Here's how the part is built. I have some questions about the finished solid (model axes, mm). Give positions to 0.01 mm unless a question says otherwise; leave off trailing zeros. Write each loop counter-clockwise with the first axis right and the second up, starting at its lowest first coordinate (ties: lowest second). Pieces come first, ordered by that corner, then holes. Notation, with made-up numbers: (76.25, 89.5) -> (110.25, 89.5) arc R23 cw to (110.25, 117.5) -> close; hole circle Ø5 at (-34, 16). An arc over 180 degrees is marked (long way). Return JSON: item names as keys, results as strings.
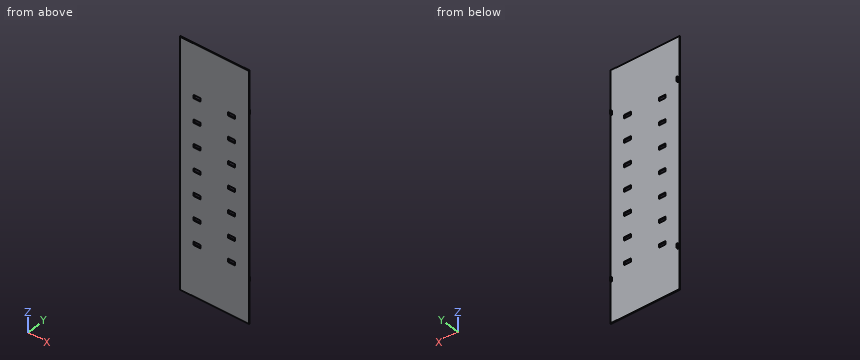
Solid Edge part; units mm, degrees
sketch "Sketch1" plane through (0, 0, 0) normal (0, -1, 0) x (1, 0, 0)
  line L0 (-254, -920.6611) -> (254, -920.6611)
  line L1 (254, -920.6611) -> (254, 920.6611)
  line L2 (254, 920.6611) -> (-254, 920.6611)
  line L3 (-254, 920.6611) -> (-254, -920.6611)
extrude "Protrusion1" add sketch "Sketch1" along normal mid plane 6.35
sketch "Sketch2" plane through (0, 3.175, 0) normal (0, 1, 0) x (-1, 0, 0)
  line L0 (-241.3, 590.4611) -> (-241.3, 622.2111)
  line L1 (-241.3, 622.2111) -> (-247.65, 622.2111)
  line L2 (-247.65, 622.2111) -> (-247.65, 590.4611)
  line L3 (-247.65, 590.4611) -> (-241.3, 590.4611)
  line L4 (241.3, 590.4611) -> (241.3, 622.2111)
  line L5 (241.3, 622.2111) -> (247.65, 622.2111)
  line L6 (247.65, 622.2111) -> (247.65, 590.4611)
  line L7 (247.65, 590.4611) -> (241.3, 590.4611)
  line L8 (-241.3, -590.4611) -> (-241.3, -622.2111)
  line L9 (-241.3, -622.2111) -> (-247.65, -622.2111)
  line L10 (-247.65, -622.2111) -> (-247.65, -590.4611)
  line L11 (-247.65, -590.4611) -> (-241.3, -590.4611)
  line L12 (241.3, -590.4611) -> (241.3, -622.2111)
  line L13 (241.3, -622.2111) -> (247.65, -622.2111)
  line L14 (247.65, -622.2111) -> (247.65, -590.4611)
  line L15 (247.65, -590.4611) -> (241.3, -590.4611)
extrude "ExtrudedProtrusion_2" add sketch "Sketch2" along normal blind 12.7 and the other way blind 0.254
sketch "Sketch3" plane through (0, -3.175, 0) normal (0, -1, 0) x (1, 0, 0)
  line L0 (-152.4, -12.7) -> (-101.6, -12.7)
  line L1 (-101.6, -12.7) -> (-101.6, 12.7)
  line L2 (-101.6, 12.7) -> (-152.4, 12.7)
  line L3 (-152.4, 12.7) -> (-152.4, -12.7)
  line L4 (-152.4, -190.5) -> (-101.6, -190.5)
  line L5 (-101.6, -190.5) -> (-101.6, -165.1)
  line L6 (-101.6, -165.1) -> (-152.4, -165.1)
  line L7 (-152.4, -165.1) -> (-152.4, -190.5)
  line L8 (-152.4, -368.3) -> (-101.6, -368.3)
  line L9 (-101.6, -368.3) -> (-101.6, -342.9)
  line L10 (-101.6, -342.9) -> (-152.4, -342.9)
  line L11 (-152.4, -342.9) -> (-152.4, -368.3)
  line L12 (-152.4, -546.1) -> (-101.6, -546.1)
  line L13 (-101.6, -546.1) -> (-101.6, -520.7)
  line L14 (-101.6, -520.7) -> (-152.4, -520.7)
  line L15 (-152.4, -520.7) -> (-152.4, -546.1)
  line L16 (-152.4, 165.1) -> (-101.6, 165.1)
  line L17 (-101.6, 165.1) -> (-101.6, 190.5)
  line L18 (-101.6, 190.5) -> (-152.4, 190.5)
  line L19 (-152.4, 190.5) -> (-152.4, 165.1)
  line L20 (-152.4, 342.9) -> (-101.6, 342.9)
  line L21 (-101.6, 342.9) -> (-101.6, 368.3)
  line L22 (-101.6, 368.3) -> (-152.4, 368.3)
  line L23 (-152.4, 368.3) -> (-152.4, 342.9)
  line L24 (-152.4, 520.7) -> (-101.6, 520.7)
  line L25 (-101.6, 520.7) -> (-101.6, 546.1)
  line L26 (-101.6, 546.1) -> (-152.4, 546.1)
  line L27 (-152.4, 546.1) -> (-152.4, 520.7)
  line L28 (152.4, -12.7) -> (101.6, -12.7)
  line L29 (101.6, -12.7) -> (101.6, 12.7)
  line L30 (101.6, 12.7) -> (152.4, 12.7)
  line L31 (152.4, 12.7) -> (152.4, -12.7)
  line L32 (152.4, -190.5) -> (101.6, -190.5)
  line L33 (101.6, -190.5) -> (101.6, -165.1)
  line L34 (101.6, -165.1) -> (152.4, -165.1)
  line L35 (152.4, -165.1) -> (152.4, -190.5)
  line L36 (152.4, -368.3) -> (101.6, -368.3)
  line L37 (101.6, -368.3) -> (101.6, -342.9)
  line L38 (101.6, -342.9) -> (152.4, -342.9)
  line L39 (152.4, -342.9) -> (152.4, -368.3)
  line L40 (152.4, -546.1) -> (101.6, -546.1)
  line L41 (101.6, -546.1) -> (101.6, -520.7)
  line L42 (101.6, -520.7) -> (152.4, -520.7)
  line L43 (152.4, -520.7) -> (152.4, -546.1)
  line L44 (152.4, 165.1) -> (101.6, 165.1)
  line L45 (101.6, 165.1) -> (101.6, 190.5)
  line L46 (101.6, 190.5) -> (152.4, 190.5)
  line L47 (152.4, 190.5) -> (152.4, 165.1)
  line L48 (152.4, 342.9) -> (101.6, 342.9)
  line L49 (101.6, 342.9) -> (101.6, 368.3)
  line L50 (101.6, 368.3) -> (152.4, 368.3)
  line L51 (152.4, 368.3) -> (152.4, 342.9)
  line L52 (152.4, 520.7) -> (101.6, 520.7)
  line L53 (101.6, 520.7) -> (101.6, 546.1)
  line L54 (101.6, 546.1) -> (152.4, 546.1)
  line L55 (152.4, 546.1) -> (152.4, 520.7)
extrude "ExtrudedCutout_1" cut sketch "Sketch3" against normal blind 225.6874
1. For pin 1 Ø7 at (x, y) = (-245, 7.5) entering from +Z; pin 2 Ø3 at (x, y) = (245.5, 10.5) entering from -Z; pin 3 Ø6 at (y, z) = (7.5, 612) entering from +X, each with a flat end and sliding along its axis, tell me the tip position at first contact or that it passes through.
Taken from the geometry:
{"pin 1": "stops at z = 622.21", "pin 2": "stops at z = -622.21", "pin 3": "stops at x = 247.65"}
2. If I drill on line 1 (X direction, y = -0.5, z = 12.5); line 2 (Y direction, x = -39.5, z = 487) (3 decimals), over which ranges is the centre line in solid material (lowest first)? Write a range as [from, to].
Taken from the geometry:
{"line 1": "x = [-254, -152.4], [-101.6, 101.6], [152.4, 254]", "line 2": "y = [-3.175, 3.175]"}
3. Suppose I cut it at B-B, the plane y = 10.5. List the corners of the cut face in (x, z) for me.
Taken from the geometry:
{"outline": "(-247.65, -622.21) -> (-241.3, -622.21) -> (-241.3, -590.46) -> (-247.65, -590.46) -> close; (-247.65, 590.46) -> (-241.3, 590.46) -> (-241.3, 622.21) -> (-247.65, 622.21) -> close; (241.3, -622.21) -> (247.65, -622.21) -> (247.65, -590.46) -> (241.3, -590.46) -> close; (241.3, 590.46) -> (247.65, 590.46) -> (247.65, 622.21) -> (241.3, 622.21) -> close"}
4. Suppose I cut it at D-D, the plane x = -189. List the corners of the cut face in (y, z) for me (3 decimals), and give its area (3 significant figures).
Taken from the geometry:
{"outline": "(-3.175, -920.661) -> (3.175, -920.661) -> (3.175, 920.661) -> (-3.175, 920.661) -> close", "area": "11,700 mm²"}
5. Suppose I cut it at C-C, the plane z = 650.5. List the corners of the cut face in (x, y) for me (3 decimals).
Taken from the geometry:
{"outline": "(-254, -3.175) -> (254, -3.175) -> (254, 3.175) -> (-254, 3.175) -> close"}
6. Suppose I cut it at A-A, the plane x = 132.5. Count the separate pieces of the cut face and the enclosed holes in it, and give its area (3 significant figures).
Taken from the geometry:
{"separate pieces": "8", "enclosed holes": "0", "area": "10,600 mm²"}
